```python
from build123d import *

# Parameters (mm, degrees)
SKETCH_1_W      = 40
SKETCH_1_H      = 40
EXTRUDE_1_DEPTH = 3.8
SKETCH_3_R      = 1
EXTRUDE_3_DEPTH = 4
SKETCH_4_R      = 1
EXTRUDE_4_DEPTH = 4


with BuildPart() as part:
    # 草图1 → 凸台-拉伸1 (new body)
    with BuildSketch(Plane.XY):
        Rectangle(SKETCH_1_W, SKETCH_1_H)
    extrude(amount=EXTRUDE_1_DEPTH)

    # 草图3 → 凸台-拉伸3 (add)
    with BuildSketch(Plane(origin=(0, 20, 0), x_dir=(1, 0, 0), z_dir=(0, 1, 0))):
        with Locations(Location((5, -1.9, 0), (0, 0, 90))):
            Circle(SKETCH_3_R)
    extrude(amount=EXTRUDE_3_DEPTH)

    # 草图4 → 凸台-拉伸4 (add)
    with BuildSketch(Plane(origin=(0, 20, 0), x_dir=(1, 0, 0), z_dir=(0, 1, 0))):
        with Locations(Location((-5, -1.9, 0), (0, 0, 90))):
            Circle(SKETCH_4_R)
    extrude(amount=EXTRUDE_4_DEPTH)


solid = part.part
```
The model under review builds one solid part; all positions refer to its coordinate system, in mm. A direction names the side the tool comes from. Round coordinates to 2 decimals unless told otherwise and drop trailing zeros. Order: outer loops, then holes, each group sorted by start corner. A loop starts at its lowest first (then second) coordinate and runs counter-clockwise, first axis right, second up. Notation, with made-up numbers: (7.5, 21.25) -> (38.5, 21.25) arc R20 ccw to (38.5, 45.25) -> close; hole circle Ø7 at (-34.75, 11.5). An arc over 180 degrees is marked (long way). Use a Markdown table: item, result.
Q1. We need section C-C on x = -1. Write out the cut boundary in (y, z), then the cut area to 3 significant figures.
Values:
| item | result |
|---|---|
| outline | (-20, 0) -> (20, 0) -> (20, 3.8) -> (-20, 3.8) -> close |
| area | 152 mm^2 |
Q2. We need section A-A on x = -5. Write out the cut boundary in (y, z).
Values:
| item | result |
|---|---|
| outline | (-20, 0) -> (20, 0) -> (20, 0.9) -> (24, 0.9) -> (24, 2.9) -> (20, 2.9) -> (20, 3.8) -> (-20, 3.8) -> close |
Q3. We need section B-B on z = 1.9. Write out the cut boundary in (x, y).
Values:
| item | result |
|---|---|
| outline | (-20, -20) -> (20, -20) -> (20, 20) -> (6, 20) -> (6, 24) -> (4, 24) -> (4, 20) -> (-4, 20) -> (-4, 24) -> (-6, 24) -> (-6, 20) -> (-20, 20) -> close |
Q4. For line 1 (Y direction, x = -2.5, z = 3.4), list the stretches that pass through material, from the lowest coordinate up.
Values:
| item | result |
|---|---|
| line 1 | y = -20 to 20 |
Q5. Tool access review of faces 4 (the cylindrical face through (4.16, 21.97, 1.36)), 5 (the flat face through (-20, 0, 2)): name each direction out of +Z, -Z, +X, -X, +Y, -Y from which nothing blocks a thin tool from reaching the whole face with its end or side.
Values:
| item | result |
|---|---|
| face 4 | +Y |
| face 5 | +Z, -Z, -X, +Y, -Y |
Q6. Clearance check with a flat-ended pin moving along its axis: P1, Ø1, axis at x = -0.5, z = 1.5, coming from the +Y side. State where the tip first meets the part, or that it passes through.
Values:
| item | result |
|---|---|
| P1 | stops at y = 20 |
Q7. Mouldability with a two-part tool opening along Z and no side actions: class faces 1 (the flat face through (0, 0, 3.8)), 2 (the cylindrical face through (-5.84, 21.97, 1.36)), 3 (the flat face through (-5, 24, 2)) as +Z half, -Z half, draft (parallel to the pull), parting line (faces both ways), or undercut.
Values:
| item | result |
|---|---|
| face 1 | +Z half |
| face 2 | parting line |
| face 3 | draft |
